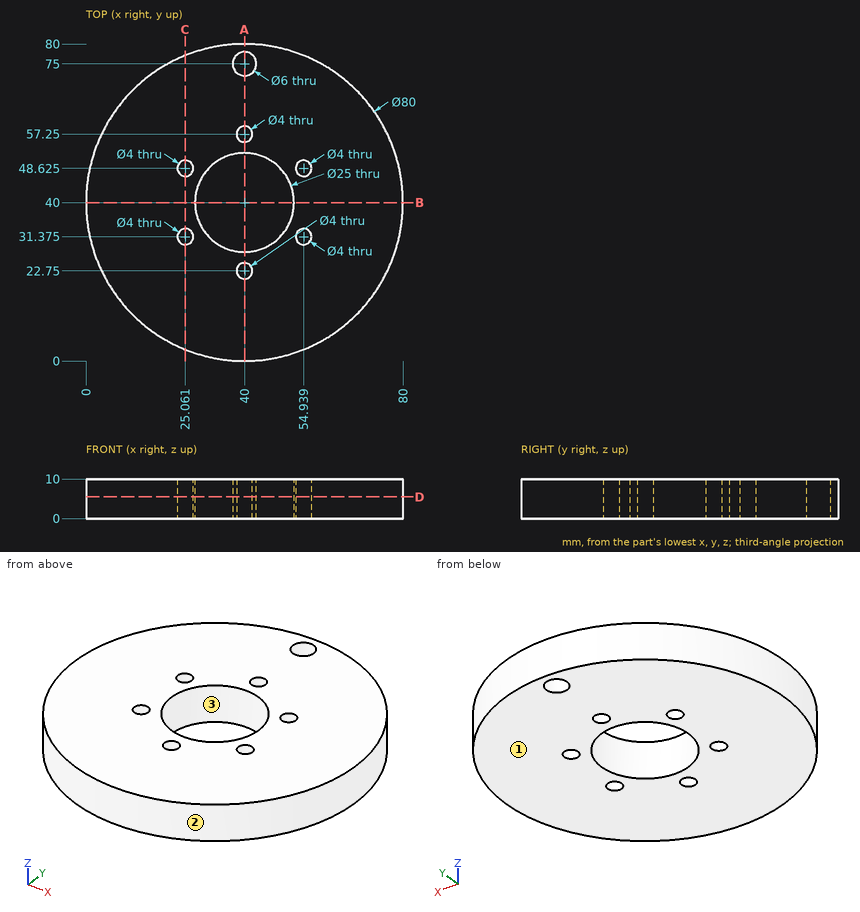
Part print with two shaded views. Sizes in mm from the minimum x, y, z corner. Round coordinates to 2 decimals unless told otherwise and drop trailing zeros. Loops run counter-clockwise (first coordinate to the right, second up) from the corner with the lowest first, then second, coordinate; pieces in that order, holes last. Notation, with made-up numbers: M 9,-16 L 15,-16 A35 ccw 15,18 Z; hole C 60.25,36.25 d4. An arc over 180 degrees is marked long. Return JSON: item names as keys, results as strings. Group by question number.
(1) Saw through at A-A, the plane x = 40. List the corners of the cut face in (y, z), and give its area (3 significant figures).
(2) Mould opens along X. For the marked faces 1, 2 and 3 say: +X half, -X half, draft (parallel to the pull), parting line (faces both ways), or undercut.
(3) Saw through at D-D, the plane z = 5.5. Give the number of separate pieces and of enclosed holes in the cut face, and give its area (3 significant figures).
(4) Saw through at B-B, the plane y = 40. List the corners of the cut face in (x, z), and give its area (3 significant figures).
(5) Wall check: probe 1 along Y at (x, z) = (40, 7); probe 2 along Y at (x, z) = (42.5, 5.25); probe 3 along X at (y, z) = (31.5, 8.5) (1 decimal). Give the ranges that are in metal, low to high. Write a range as [from, to].
(6) Drop flat-ended pins along their axis: P1, Ø3, axis at x = 57.5, z = 5, coming from the +Y side; P2, Ø5, axis at x = 28.5, z = 6.5, coming from the -Y side; P3, Ø3.5, axis at x = 25.06, y = 31.38, coming from the +Z side; P4, Ø5, axis at x = 64.5, z = 2.5, coming from the -Y side. Give the stop position or say it passes through.
(7) Saw through at C-C, the plane x = 25. List the corners of the cut face in (y, z), and give its area (3 significant figures).
Answer list:
{
 "1": {"outline": "M 0,0 L 20.75,0 L 20.75,10 L 0,10 Z; M 24.75,0 L 27.5,0 L 27.5,10 L 24.75,10 Z; M 52.5,0 L 55.25,0 L 55.25,10 L 52.5,10 Z; M 59.25,0 L 72,0 L 72,10 L 59.25,10 Z; M 78,0 L 80,0 L 80,10 L 78,10 Z", "area": "410 mm2"},
 "2": {"face 1": "draft", "face 2": "parting line", "face 3": "undercut"},
 "3": {"separate pieces": "1", "enclosed holes": "8", "area": "4,430 mm2"},
 "4": {"outline": "M 0,0 L 27.5,0 L 27.5,10 L 0,10 Z; M 52.5,0 L 80,0 L 80,10 L 52.5,10 Z", "area": "550 mm2"},
 "5": {"probe 1": "[0, 20.75], [24.75, 27.5], [52.5, 55.25], [59.25, 72], [78, 80]", "probe 2": "[0.08, 27.75], [52.25, 73.34], [76.66, 79.92]", "probe 3": "[0.9, 23.1], [27.1, 30.8], [49.2, 52.9], [56.9, 79.1]"},
 "6": {"P1": "y = 76.66", "P2": "y = 1.03", "P3": "through", "P4": "y = 6.59"},
 "7": {"outline": "M 2.92,0 L 29.38,0 L 29.38,10 L 2.92,10 Z; M 33.37,0 L 46.63,0 L 46.63,10 L 33.37,10 Z; M 50.62,0 L 77.08,0 L 77.08,10 L 50.62,10 Z", "area": "662 mm2"}
}
